```python
from build123d import *

# Parameters (mm, degrees)
F1_DEPTH = 1.5
F2_R     = 1.524
F3_DEPTH = 25
F5_R     = 10
F6_DEPTH = 12
F7_W     = 3
F7_H     = 3
F8_DEPTH = 2
F9_SIZE  = 1


with BuildPart() as f1:
    # F0 (on Top) → F1 (new body)
    with BuildSketch(Plane.XY):
        Polygon((12.7, -2), (12.7, -6.35), (41.148, -6.35), (41.148, -2), (43.148, 0), (53.848, 0), (53.848, 44.45), (0, 44.45), (0, 0), (10.7, 0), align=None)
    extrude(amount=F1_DEPTH)

    # F2 (on face) → F3 (cut)
    with BuildSketch(Plane.XY.offset(1.5)):
        with Locations((3.175, 41.275)):
            Circle(F2_R)
        with Locations((50.673, 41.275)):
            Circle(F2_R)
        with Locations((16.51, -3.175)):
            Circle(F2_R)
        with Locations((37.338, -3.175)):
            Circle(F2_R)
    extrude(amount=-F3_DEPTH, mode=Mode.SUBTRACT)

    # F5 (on face) → F6 (join)
    with BuildSketch(Plane.XY.offset(1.5)):
        with Locations((26.924, 29.45)):
            Circle(F5_R)
    extrude(amount=F6_DEPTH)

    # F7 (on face) → F8 (join)
    with BuildSketch(Plane.XY.offset(1.5)):
        with Locations((26.924, -1.85)):
            Rectangle(F7_W, F7_H)
    extrude(amount=F8_DEPTH)

    # F9
    f9_edges = [f1.edges().sort_by_distance(p)[0] for p in [
        (26.924, -0.35, 3.5),
        (25.424, -1.85, 3.5),
        (28.424, -1.85, 3.5),
        (26.924, -3.35, 3.5),
    ]]
    chamfer(f9_edges, length=F9_SIZE)


solid = f1.part
```
Build history of the part. All positions in model axes, mm. A direction names the side the tool comes from. Round coordinates to 2 decimals unless told otherwise and drop trailing zeros. Write each loop counter-clockwise with the first axis right and the second up, starting at its lowest first coordinate (ties: lowest second). Pieces come first, ordered by that corner, then holes. Notation, with made-up numbers: (68, 8.5) -> (76, 8.5) arc R14 ccw to (76, 25.5) -> close; hole circle Ø6 at (60, 55.25). An arc over 180 degrees is marked (long way). Put each result on its own line as item: value.
Item 1: Flat gauge pins, fed straight in: P1, Ø4, axis at x = 3.175, y = 41.275, coming from the +Z side; P2, Ø8, axis at x = 14.5, z = 2, coming from the +Y side; P3, Ø0.8, axis at x = 27, z = 2, coming from the +Y side; P4, Ø1.2, axis at x = 5.5, z = 1, coming from the -Y side. Where does each tip first touch, or does it go through?
Here are the results:
P1: stops at z = 1.5
P2: stops at y = 44.45
P3: stops at y = 39.45
P4: stops at y = 0
Item 2: Tool access for faces 1 (the face through (12.7, -4, 1)), 2 (the face through (25.622, 39.365, 7.416)), 3 (the face through (41.148, -4, 1)): list every direction of +Z, -Z, +X, -X, +Y, -Y with a clear straight run to the whole face (end or side of a thin tool).
Here are the results:
face 1: +Z, -Z, -X, -Y
face 2: +Z
face 3: +Z, -Z, +X, -Y
Item 3: Wall check: probe 1 along Y at (x, z) = (16.51, 0.8); probe 2 along Z at (x, y) = (37.5, 5); probe 3 along X at (y, z) = (27, 2.5). Give the ranges that are in metal, low to high. Write a range as from..to.
Here are the results:
probe 1: y = -6.35..-4.7, -1.65..44.45
probe 2: z = 0..1.5
probe 3: x = 17.23..36.62
Item 4: Slice it at D-D, the plane y = 17. Give the cut face in (x, z), plus the area to 3 significant figures.
Here are the results:
outline: (0, 0) -> (53.85, 0) -> (53.85, 1.5) -> (0, 1.5) -> close
area: 80.8 mm^2
Item 5: Slice it at A-A, the plane y = 29.45. Give the cut face in (x, z).
Here are the results:
outline: (0, 0) -> (53.85, 0) -> (53.85, 1.5) -> (36.92, 1.5) -> (36.92, 13.5) -> (16.92, 13.5) -> (16.92, 1.5) -> (0, 1.5) -> close
Item 6: Slice it at C-C, the plane z = 7.5. Give the cut face in (x, y), plus the area to 3 significant figures.
Here are the results:
outline: circle Ø20 at (26.92, 29.45)
area: 314 mm^2
Item 7: Slice it at B-B, the plane x = 24.5. Give the cut face in (y, z), plus the area to 3 significant figures.
Here are the results:
outline: (-6.35, 0) -> (44.45, 0) -> (44.45, 1.5) -> (39.15, 1.5) -> (39.15, 13.5) -> (19.75, 13.5) -> (19.75, 1.5) -> (-6.35, 1.5) -> close
area: 309 mm^2
